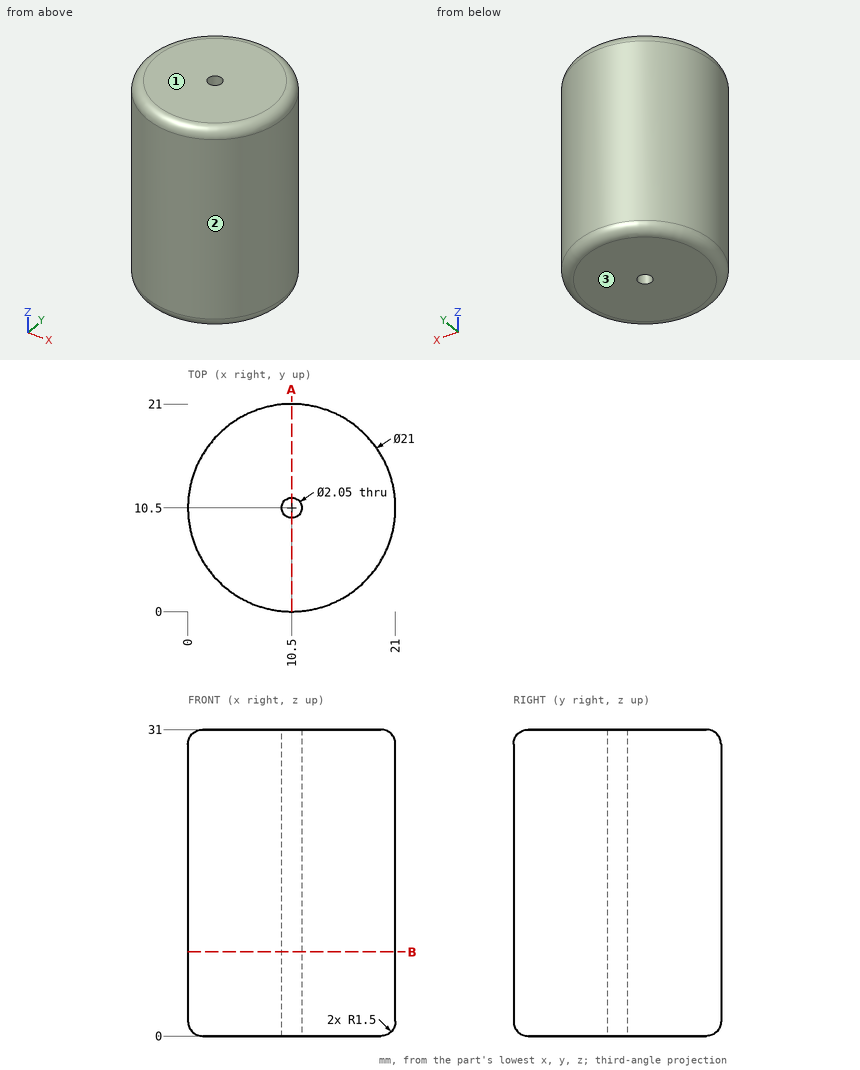
Part print with two shaded views. Sizes in mm from the minimum x, y, z corner. Coordinates: 2 decimals unless noted, no trailing zeros. Write each loop counter-clockwise with the first axis right and the second up, starting at its lowest first coordinate (ties: lowest second). Pieces come first, ordered by that corner, then holes. Notation, with made-up numbers: (-26, 58.25) -> (28, 58.25) arc R28 cw to (28, 81.25) -> close; hole circle Ø11 at (14, -15). An arc over 180 degrees is marked (long way). Return JSON: item names as keys, results as strings. Group by question number.
Q1. Cut at A-A, the plane x = 10.5. Give the cut face in (y, z) (3 decimals), then the cut area to 3 significant figures.
Q2. Drill centre lines: line 1 (Y direction, x = 10.5, z = 17.5) (3 decimals); line 2 (Y direction, x = 5.5, z = 30); line 3 (Y direction, x = 19, z = 26). Where is each one in solid material? Low to high.
Q3. Flat gauge pins, fed straight in: pin 1 (6 mm diameter, centred on y = 4, z = 7, fed in from +X); pin 2 (1.8 mm diameter, centred on x = 10.5, y = 10.5, fed in from +Z); pin 3 (1.5 mm diameter, centred on x = 7.5, z = 19, fed in from +Y). Where does each tip first touch, or does it go through?
Q4. Cut at B-B, the plane z = 8.5. Give the cut face in (x, y) (3 decimals), then the cut area to 3 significant figures.
Q5. Pull direction Z, two halves, no side cores. Call the marked faces 1, 2 and 3: released by +Z, released by -Z, zero draft, split by the parting line, or undercut.
Returned:
{
 "1": {"outline": "(0, 1.5) arc R1.5 ccw to (1.5, 0) -> (9.475, 0) -> (9.475, 31) -> (1.5, 31) arc R1.5 ccw to (0, 29.5) -> close; (11.525, 0) -> (19.5, 0) arc R1.5 ccw to (21, 1.5) -> (21, 29.5) arc R1.5 ccw to (19.5, 31) -> (11.525, 31) -> close", "area": "586 mm2"},
 "2": {"line 1": "y = 0 to 9.475, 11.525 to 21", "line 2": "y = 1.36 to 19.64", "line 3": "y = 4.34 to 16.66"},
 "3": {"pin 1": "stops at x = 20.4", "pin 2": "passes through", "pin 3": "stops at y = 20.76"},
 "4": {"outline": "circle Ø21 at (10.5, 10.5); hole circle Ø2.05 at (10.5, 10.5)", "area": "343 mm2"},
 "5": {"face 1": "released by +Z", "face 2": "zero draft", "face 3": "released by -Z"}
}
